Source: three-view drawing plus pictorial views. Frame: mm from the lowest corner of the part. Give positions to 0.01 mm unless a question says otherwise; leave off trailing zeros. Loops run counter-clockwise (first coordinate to the right, second up) from the corner with the lowest first, then second, coordinate; pieces in that order, holes last.
1. Draft query along X for the marked faces 1, 2 and 3. Return one class per face: +X half, -X half, draft (parallel to the pull), parting line (faces both ways), or undercut.
2. Section C-C, the plane z = 79. Output: boundary loops of the cut face in (x, y).
3. First-contact query: P1, Ø3, axis at x = 31.5, y = 26, coming from the -Z side; P2, Ø4, axis at y = 29, z = 35, coming from the +X side; P3, Ø12, axis at x = 16, z = 69, coming from the +Y side; P4, Ø5, axis at x = 11.5, z = 36.5, coming from the -Y side. Flat tips, straight axial feed; report the tip coordinate or a pass-through.
4. Section A-A, the plane y = 18.5. Output: boundary loops of the cut face in (x, z).
5. Material intervals for line 1 along Y through (x, z) = (18.5, 102); line 2 along X through (y, z) = (18, 103); line 3 along Z through (x, y) = (27, 21), sorted ascending.
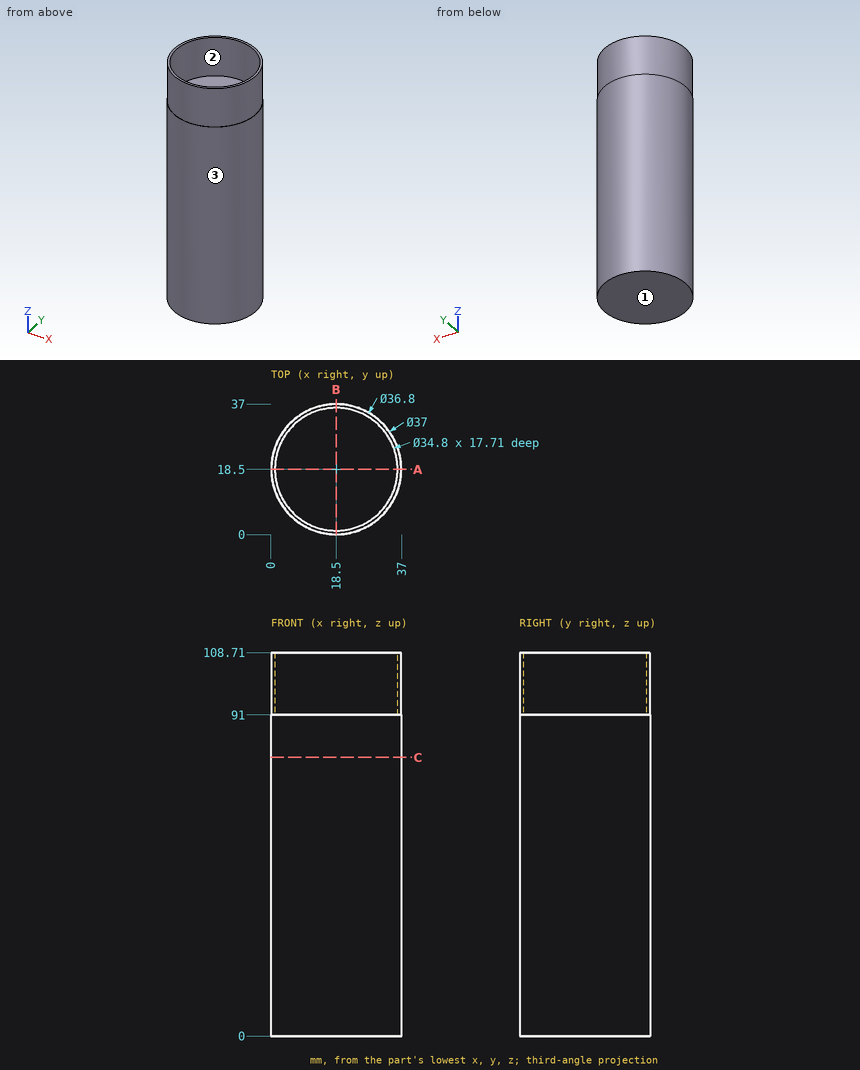
Answers below:
1. face 1: draft
1. face 2: undercut
1. face 3: parting line
2. outline: circle Ø37 at (18.5, 18.5)
3. P1: stops at z = 0
3. P2: stops at x = 34.93
3. P3: stops at y = 37
3. P4: stops at y = 0.56
4. outline: (0, 0) - (37, 0) - (37, 91) - (36.9, 91) - (36.9, 108.71) - (35.9, 108.71) - (35.9, 91) - (1.1, 91) - (1.1, 108.71) - (0.1, 108.71) - (0.1, 91) - (0, 91) - close
5. line 1: y = 0.1 to 1.1, 35.9 to 36.9
5. line 2: x = 0.11 to 1.11, 35.89 to 36.89
5. line 3: z = 0 to 91
